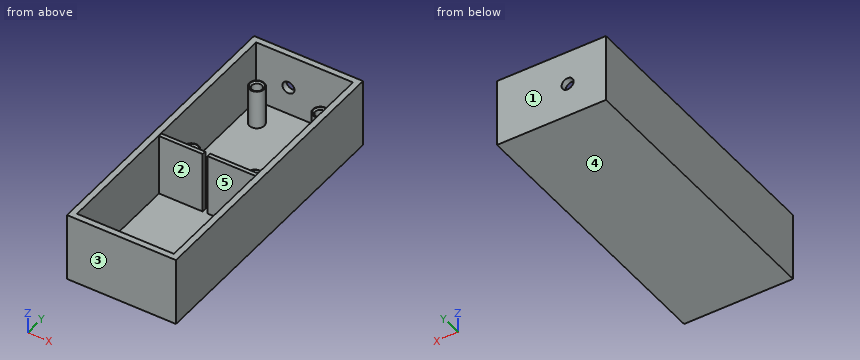
from build123d import *

# Parameters (mm, degrees)
SKETCH1_W                            = 45.72
SKETCH1_H                            = 119.38
BOSS_EXTRUDE1_DEPTH                  = 14.403566373
SHELL3_T                             = -2.54
SKETCH4_R                            = 3.175
BOSS_EXTRUDE2_DEPTH                  = 16.51
F_8_0_199_DIAMETER_HOLE1_D           = 5.0546
F_8_0_199_DIAMETER_HOLE1_DEPTH       = 2.54
SKETCH19_W                           = 40.64
SKETCH19_H                           = 1.642675469
BOSS_EXTRUDE3_DEPTH                  = 25.908
SKETCH23_W                           = 2.002221862
SKETCH23_H                           = 25.908
CUT_EXTRUDE2_DEPTH                   = 15.748
F_4_0_209_DIAMETER_HOLE1_D           = 4.2926
F_4_0_209_DIAMETER_HOLE1_DEPTH       = 13.462
F_4_0_209_DIAMETER_HOLE1_CSINK_D     = 5.6896
F_4_0_209_DIAMETER_HOLE1_CSINK_ANGLE = 100
F_4_0_209_DIAMETER_HOLE1_TIP         = 1.289627147


with BuildPart() as part:
    # Sketch1 → Boss-Extrude1 (new body, symmetric)
    with BuildSketch(Plane.XY):
        Rectangle(SKETCH1_W, SKETCH1_H)
    extrude(amount=BOSS_EXTRUDE1_DEPTH, both=True)

    # Shell3
    shell3_openings = [part.faces().sort_by_distance(p)[0] for p in [
        (0, 0, 14.403566373),
    ]]
    offset(amount=SHELL3_T, openings=shell3_openings, kind=Kind.INTERSECTION)

    # Sketch4 → Boss-Extrude2 (add)
    with BuildSketch(Plane.XY.offset(-11.863566373)):
        with Locations((-13.335, 46.99)):
            Circle(SKETCH4_R)
        with Locations((13.335, 46.99)):
            Circle(SKETCH4_R)
        with Locations((13.335, 5.08)):
            Circle(SKETCH4_R)
        with Locations((-13.335, 5.08)):
            Circle(SKETCH4_R)
    extrude(amount=BOSS_EXTRUDE2_DEPTH)

    # #8 (0.199) Diameter Hole1
    with Locations(Plane(origin=(0, 59.69, 0), x_dir=(1, 0, 0), z_dir=(0, 1, 0))):
        with Locations((-6.761861897, 0), (-42.285600541, -5.559615493)):
            Hole(F_8_0_199_DIAMETER_HOLE1_D / 2, depth=F_8_0_199_DIAMETER_HOLE1_DEPTH)

    # Sketch19 → Boss-Extrude3 (add)
    with BuildSketch(Plane.XY.offset(-11.863566373)):
        with Locations((0, -3.991920643)):
            Rectangle(SKETCH19_W, SKETCH19_H)
    extrude(amount=BOSS_EXTRUDE3_DEPTH)

    # Sketch23 → Cut-Extrude2 (cut)
    with BuildSketch(Plane.XZ.offset(4.813258377)):
        with Locations((-1.001110931, 1.090433627)):
            Rectangle(SKETCH23_W, SKETCH23_H)
    extrude(amount=-CUT_EXTRUDE2_DEPTH, mode=Mode.SUBTRACT)

    # #4 (0.209) Diameter Hole1
    with Locations(Plane.XY.offset(4.646433627)):
        with Locations((-13.335, 5.08), (-13.335, 46.99), (13.335, 5.08), (13.335, 46.99)):
            CounterSinkHole(F_4_0_209_DIAMETER_HOLE1_D / 2, F_4_0_209_DIAMETER_HOLE1_CSINK_D / 2, depth=F_4_0_209_DIAMETER_HOLE1_DEPTH, counter_sink_angle=F_4_0_209_DIAMETER_HOLE1_CSINK_ANGLE)
            with Locations((0, 0, -(F_4_0_209_DIAMETER_HOLE1_DEPTH + F_4_0_209_DIAMETER_HOLE1_TIP / 2))):  # 118° drill point
                Cone(0, F_4_0_209_DIAMETER_HOLE1_D / 2, F_4_0_209_DIAMETER_HOLE1_TIP, mode=Mode.SUBTRACT)


solid = part.part
Check sheet for the modelled part. Datum: model origin and axes. Units: mm. Face numbers are marked on the shaded views. A direction names the side the tool comes from. Coordinates: 2 decimals unless noted, no trailing zeros. Loops run counter-clockwise (first coordinate to the right, second up) from the corner with the lowest first, then second, coordinate; pieces in that order, holes last. Notation, with made-up numbers: (18.25, 66) -> (34.25, 66) arc R28 ccw to (34.25, 98) -> close; hole circle Ø3 at (72, 12). An arc over 180 degrees is marked (long way). Write item = value, one per line. Start each with the question number.
1. Depth check by flat-ended pin: P1, Ø4, axis at x = 13.335, y = 5.08, coming from the +Z side; P2, Ø7, axis at x = -14.5, y = 5.5, coming from the +Z side; P3, Ø0.8, axis at x = 6, y = -4.5, coming from the +Z side; P4, Ø1.5, axis at x = -8.5, z = 1, coming from the +Y side. Enter the tip coordinate at first touch or a pass-through.
2. Tool access check on the marked faces 4 and 5. Record the directions out of +Z, -Z, +X, -X, +Y, -Y that give a thin tool (end or side, any length) a straight path to the whole face; none if there is none.
3. Draft check along Y on the marked faces 1, 2 and 3. Enter one of: released by +Y, released by -Y, zero draft, split by the parting line, or undercut.
4. Section check C-C on x = -6. Record the cut outline in (y, z), then the cut area to 3 significant figures.
5. Section check D-D on y = 14.5. Record the cut outline in (x, z).
6. Section check B-B on z = 6. Record the cut outline in (x, y), then the cut area to 3 significant figures.
7. Material ranges on line 1 (Y direction, x = 14, z = 7); line 2 (Y direction, x = -6.5, z = 2.25); line 3 (X direction, y = 43.5, z = -10.5), recorded low to high.
8. Section check A-A on z = 0. Give the number of separate pieces and of enclosed holes in the cut face, then the cut area to 3 significant figures.
Responses:
q1.P1 = -8.9
q1.P2 = 4.65
q1.P3 = 14.04
q1.P4 = 59.69
q2.face_4 = -Z, +X, -X, +Y, -Y
q2.face_5 = +Z
q3.face_1 = released by +Y
q3.face_2 = undercut
q3.face_3 = released by -Y
q4.outline = (-59.69, -14.4) -> (59.69, -14.4) -> (59.69, -2.41) -> (57.15, -2.41) -> (57.15, -11.86) -> (-3.17, -11.86) -> (-3.17, 14.04) -> (-4.81, 14.04) -> (-4.81, -11.86) -> (-57.15, -11.86) -> (-57.15, 14.4) -> (-59.69, 14.4) -> close; (57.15, 2.41) -> (59.69, 2.41) -> (59.69, 14.4) -> (57.15, 14.4) -> close
q4.area = 467 mm2
q5.outline = (-22.86, -14.4) -> (22.86, -14.4) -> (22.86, 14.4) -> (20.32, 14.4) -> (20.32, -11.86) -> (-20.32, -11.86) -> (-20.32, 14.4) -> (-22.86, 14.4) -> close
q6.outline = (-22.86, -59.69) -> (22.86, -59.69) -> (22.86, 59.69) -> (-22.86, 59.69) -> close; hole (-20.32, -57.15) -> (20.32, -57.15) -> (20.32, -4.81) -> (0, -4.81) -> (0, -3.17) -> (20.32, -3.17) -> (20.32, 57.15) -> (-20.32, 57.15) -> (-20.32, -3.17) -> (-2, -3.17) -> (-2, -4.81) -> (-20.32, -4.81) -> close
q6.area = 876 mm2
q7.line_1 = -59.69 to -57.15, -4.81 to -3.17, 57.15 to 59.69
q7.line_2 = -59.69 to -57.15, -4.81 to -3.17
q7.line_3 = -22.86 to -20.32, 20.32 to 22.86
q8.separate_pieces = 5
q8.enclosed_holes = 4
q8.area = 932 mm2
